```python
from build123d import *

# Parameters (mm, degrees)
F0_W     = 1400
F0_H     = 180
F1_DEPTH = 220
F2_W     = 1394
F2_H     = 174
F3_DEPTH = 217
F4_R     = 15
F5_DEPTH = 3


with BuildPart() as f1:
    # F0 (on Top) → F1 (new body)
    with BuildSketch(Plane.XY):
        with Locations((653.785665, 53.946961)):
            Rectangle(F0_W, F0_H)
    extrude(amount=F1_DEPTH)

    # F2 (on face) → F3 (cut)
    with BuildSketch(Plane.XY.offset(220)):
        with Locations((653.785665, 53.946961)):
            Rectangle(F2_W, F2_H)
    extrude(amount=-F3_DEPTH, mode=Mode.SUBTRACT)

    # F4 (on face) → F5 (cut, through all)
    with BuildSketch(Plane.XZ.offset(36.053039)):
        with Locations((553.785665, 175)):
            Circle(F4_R)
        with Locations((1059.785665, 175)):
            Circle(F4_R)
    extrude(amount=-F5_DEPTH, mode=Mode.SUBTRACT)


solid = f1.part
```
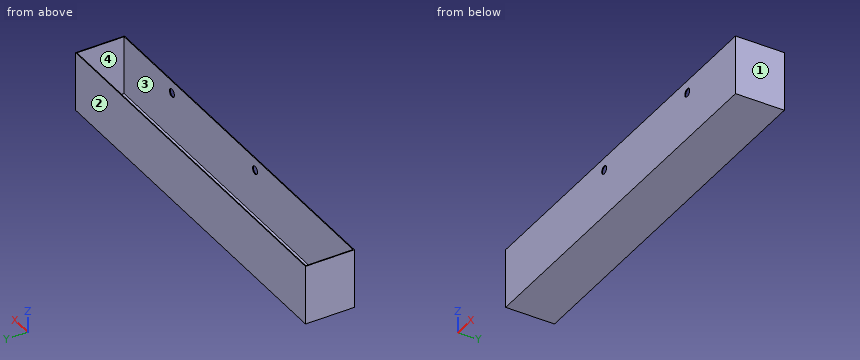
The listing builds one solid part. Answer for the finished solid, in the listing's coordinates (mm). Face numbers are marked on the shaded views. Give positions to 0.01 mm unless a question says otherwise; leave off trailing zeros. Order: outer loops, then holes, each group sorted by start corner. A loop starts at its lowest first (then second) coordinate and runs counter-clockwise, first axis right, second up. Notation, with made-up numbers: M 39,11 L 79,11 A23 ccw 79,37 Z; hole C 89,23 d5. An arc over 180 degrees is marked long. Put each result on its own line as item: value. Start each with the question number.
Item 1: The part is cut by section C-C, the plane z = 104. Determine the outline of the cut face in (x, y), and give its area (3 significant figures).
Item 2: The part is cut by section A-A, the plane z = 175. Determine the outline of the cut face in (x, y).
Item 3: For a pull along Y with two mould halves and no side action, classify the marked faces 1, 2, 3 and 4 as +Y half, -Y half, draft (parallel to the pull), parting line (faces both ways), or undercut.
Item 4: Find the intervals of material crossed by line 1 along Y through (x, z) = (1085, 39.5); line 2 along X through (y, z) = (90.5, 163); line 3 along Z through (x, y) = (37.5, -7.5), in increasing order.
Item 5: The part is cut by section B-B, the plane y = 6. Determine the outline of the cut face in (x, z).
Item 6: The part is cut by section D-D, the plane x = 321.5. Determine the outline of the cut face in (y, z).
Item 7: Flat-ended cylindrical pins translate along their axes: P1, Ø4, axis at x = 380.5, y = 96, coming from the -Z side; P2, Ø6, axis at x = 506, y = 29, coming from the +Z side. Find the tip coordinate at first contact, or state that the pin passes through.
Answer key:
1. outline: M -46.21,-36.05 L 1353.79,-36.05 L 1353.79,143.95 L -46.21,143.95 Z; hole M -43.21,-33.05 L 1350.79,-33.05 L 1350.79,140.95 L -43.21,140.95 Z
1. area: 9,440 mm²
2. outline: M -46.21,-36.05 L 538.79,-36.05 L 538.79,-33.05 L -43.21,-33.05 L -43.21,140.95 L 1350.79,140.95 L 1350.79,-33.05 L 1074.79,-33.05 L 1074.79,-36.05 L 1353.79,-36.05 L 1353.79,143.95 L -46.21,143.95 Z; M 568.79,-36.05 L 1044.79,-36.05 L 1044.79,-33.05 L 568.79,-33.05 Z
3. face 1: draft
3. face 2: +Y half
3. face 3: undercut
3. face 4: undercut
4. line 1: y = -36.05 to -33.05, 140.95 to 143.95
4. line 2: x = -46.21 to -43.21, 1350.79 to 1353.79
4. line 3: z = 0 to 3
5. outline: M -46.21,0 L 1353.79,0 L 1353.79,220 L 1350.79,220 L 1350.79,3 L -43.21,3 L -43.21,220 L -46.21,220 Z
6. outline: M -36.05,0 L 143.95,0 L 143.95,220 L 140.95,220 L 140.95,3 L -33.05,3 L -33.05,220 L -36.05,220 Z
7. P1: stops at z = 0
7. P2: stops at z = 3
